Build history of the part. All positions in model axes, mm. Face numbers are marked on the shaded views. A direction names the side the tool comes from. Give positions to 0.01 mm unless a question says otherwise; leave off trailing zeros. Write each loop counter-clockwise with the first axis right and the second up, starting at its lowest first coordinate (ties: lowest second). Pieces come first, ordered by that corner, then holes. Notation, with made-up numbers: (-11, 61.5) -> (32, 61.5) arc R10 ccw to (32, 72.5) -> close; hole circle Ø6 at (59.25, -13). An arc over 180 degrees is marked (long way). Write item = value, one per line. Start each with the question number.
Q1. Drop a flat-ended pin along its axis: P1, Ø2, axis at y = -4.5, z = 1, coming from the +X side. Give the stop position or say it passes through.
Q2. Saw through at D-D, the plane x = 4.75. List the corners of the cut face in (y, z), then the cut area to 3 significant figures.
Q3. Saw through at C-C, the plane y = -3. List the corners of the cut face in (x, z), then the cut area to 3 significant figures.
Q4. Mould opens along Z. For the marked faces 1, 2 and 3 say: pulls with the +Z half, pulls with the -Z half, needs draft (parallel to the pull), parting line crosses it, or undercut.
Q5. Wall check: line 1 (Z direction, x = -1.5, y = -8.5); line 2 (X direction, y = -1.5, z = -0.5); line 3 (Z direction, x = 2.5, y = -5.75). Give the ranges that are in metal, low to high.
Q6. Saw through at B-B, the plane z = -0.75. List the corners of the cut face in (x, y).
Q7. Tool access for the marked faces 4 and 5: list every direction of +Z, -Z, +X, -X, +Y, -Y with a clear straight run to the whole face (end or side of a thin tool).
Q8. Saw through at A-A, the plane x = 1.5. List the corners of the cut face in (y, z), then the cut area to 3 significant figures.
from build123d import *

# Parameters (mm, degrees)
PAD_DEPTH = 10


with BuildPart() as part:
    # Sketch (on XZ_Plane of Origin) → Pad (new body)
    with BuildSketch(Plane.XZ):
        with BuildLine():
            Line((-2.45, 0.55), (-2.45, -0.55))
            ThreePointArc((-2.45, -0.55), (-2.303553, -0.903553), (-1.95, -1.05))
            Line((-1.95, -1.05), (1.95, -1.05))
            Line((3.25, -1.05), (1.95, -1.05))
            ThreePointArc((3.25, -1.05), (3.603553, -0.903553), (3.75, -0.55))
            ThreePointArc((5.75, -0.55), (4.75, 0.45), (3.75, -0.55))
            ThreePointArc((3.25, -3.05), (5.017767, -2.317767), (5.75, -0.55))
            Line((1.95, -3.05), (3.25, -3.05))
            Line((-1.95, -3.05), (1.95, -3.05))
            ThreePointArc((-4.45, -0.55), (-3.717767, -2.317767), (-1.95, -3.05))
            Line((-4.45, 0.55), (-4.45, -0.55))
            ThreePointArc((-1.95, 3.05), (-3.717767, 2.317767), (-4.45, 0.55))
            Line((1.95, 3.05), (-1.95, 3.05))
            ThreePointArc((2.45, 2.55), (2.303553, 2.903553), (1.95, 3.05))
            Line((2.45, 2.55), (2.45, 1.55))
            ThreePointArc((1.95, 1.05), (2.303553, 1.196447), (2.45, 1.55))
            Line((1.95, 1.05), (-1.95, 1.05))
            ThreePointArc((-1.95, 1.05), (-2.303553, 0.903553), (-2.45, 0.55))
        make_face()
    extrude(amount=PAD_DEPTH)


solid = part.part
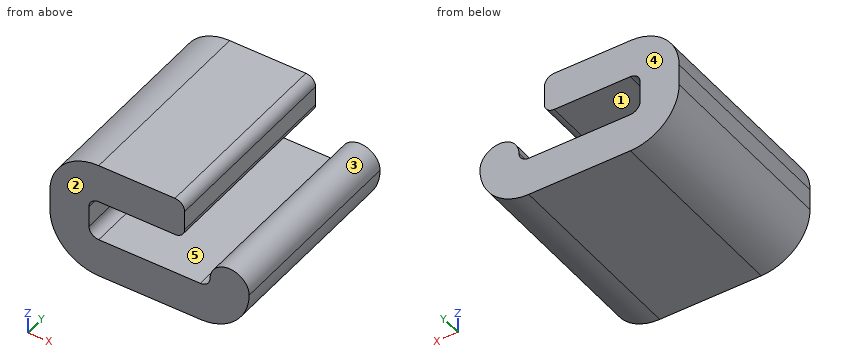
Report:
q1.P1 = 5.59
q2.outline = (-10, -2.55) -> (0, -2.55) -> (0, 0.45) -> (-10, 0.45) -> close
q2.area = 30.0 mm2
q3.outline = (-4.45, -0.55) arc R2.5 ccw to (-1.95, -3.05) -> (3.25, -3.05) arc R2.5 ccw to (5.75, -0.55) arc R1 ccw to (3.75, -0.55) arc R0.5 cw to (3.25, -1.05) -> (-1.95, -1.05) arc R0.5 cw to (-2.45, -0.55) -> (-2.45, 0.55) arc R0.5 cw to (-1.95, 1.05) -> (1.95, 1.05) arc R0.5 ccw to (2.45, 1.55) -> (2.45, 2.55) arc R0.5 ccw to (1.95, 3.05) -> (-1.95, 3.05) arc R2.5 ccw to (-4.45, 0.55) -> close
q3.area = 37.0 mm2
q4.face_1 = undercut
q4.face_2 = needs draft
q4.face_3 = pulls with the +Z half
q5.line_1 = -3.05 to -1.05, 1.05 to 3.05
q5.line_2 = -4.45 to -2.45, 3.75 to 5.75
q5.line_3 = -3.05 to -1.05
q6.outline = (-4.44, -10) -> (-2.41, -10) -> (-2.41, 0) -> (-4.44, 0) -> close; (3.71, -10) -> (5.74, -10) -> (5.74, 0) -> (3.71, 0) -> close
q7.face_4 = +Z, -Z, +X, -X, +Y
q7.face_5 = +Y, -Y
q8.outline = (-10, -3.05) -> (0, -3.05) -> (0, -1.05) -> (-10, -1.05) -> close; (-10, 1.05) -> (0, 1.05) -> (0, 3.05) -> (-10, 3.05) -> close
q8.area = 40.0 mm2
